Could you check a few things on this model? Use its own coordinates, in mm. A direction names the side the tool comes from. Give positions to 0.01 mm unless a question says otherwise; leave off trailing zeros. Loops run counter-clockwise (first coordinate to the right, second up) from the corner with the lowest first, then second, coordinate; pieces in that order, holes last.
1. Imagine slicing it at A-A (x = 0). List the corners of the cut face in (y, z) for me.
2. Imagine slicing it at C-C (z = 25). List the corners of the cut face in (x, y) for me.
3. Imagine slicing it at B-B (y = 3.5). List the corners of the cut face in (x, z) for me, plus the area to 3 significant figures.
4. Thinking about a two-plate mould opening in Z: for faces 1 (the cylindrical face through (14.531, 8.972, -15.846)), 2 (the cylindrical face through (-27.53, 4.82, -0.33)), 3 (the flat face through (-17.4, 11, 3.1)), which applies, +Z half, -Z half, draft (parallel to the pull), parting line (faces both ways), or undercut?
5. For P1, Ø6.5, axis at x = -25, z = 0, coming from the +Y side; P2, Ø21, axis at x = 0, z = 0, coming from the +Y side; P3, Ø5, axis at x = 17.5, z = 18, coming from the -Y side; P4, Ø6, axis at x = -11, y = 1.5, coming from the +Z side, each with a flat end and sliding along its axis, tell me the tip position at first contact or that it passes through.
6. I need wall thicknesses on line 1 along X through (y, z) = (5.75, 0); line 2 along X through (y, z) = (8.5, 0); line 3 along Y through (x, z) = (13, -19). Which ranges of each line are inside material? Lowest first, please.
7. Imagine slicing it at D-D (x = -11). List the corners of the cut face in (y, z) for me.
8. For faces 4 (the flat face through (-9, 7, 20)), 5 (the cylindrical face through (27.53, 4.82, 0.33)), which set-ups out of +Z, -Z, +X, -X, +Y, -Y let a thin tool reach every point of the face, with its end or its side?
```python
from build123d import *

# Parameters (mm, degrees)
SKETCH1_R                    = 30
SKETCH1_R_2                  = 17.5
BOSS_EXTRUDE1_DEPTH          = 7
SKETCH2_R                    = 21.5
SKETCH2_R_2                  = 17.5
BOSS_EXTRUDE2_DEPTH          = 4
SKETCH4_R                    = 2.55
CUT_EXTRUDE1_DEPTH           = 44.829214002
CHAMFER1_SIZE                = 2.7
CIRPATTERN1_COUNT            = 4
CHAMFER1_OF_CIRPATTERN1_SIZE = 2.7


with BuildPart() as part:
    # Sketch1 → Boss-Extrude1 (new body)
    with BuildSketch(Plane(origin=(0, 0, 0), x_dir=(1, 0, 0), z_dir=(0, 1, 0))):
        with Locations(Location((0, 0, 0), (0, 0, 270))):
            Circle(SKETCH1_R)
        with Locations(Location((0, 0, 0), (0, 0, 270))):
            Circle(SKETCH1_R_2, mode=Mode.SUBTRACT)
    extrude(amount=BOSS_EXTRUDE1_DEPTH)

    # Sketch2 → Boss-Extrude2 (add)
    with BuildSketch(Plane(origin=(0, 7, 0), x_dir=(1, 0, 0), z_dir=(0, 1, 0))):
        with Locations(Location((0, 0, 0), (0, 0, 270))):
            Circle(SKETCH2_R)
        with Locations(Location((0, 0, 0), (0, 0, 270))):
            Circle(SKETCH2_R_2, mode=Mode.SUBTRACT)
    extrude(amount=BOSS_EXTRUDE2_DEPTH)

    # Sketch4 → Cut-Extrude1 (cut, through all)
    with BuildSketch(Plane.XZ):
        with Locations(Location((25, 0, 0), (0, 0, 270))):
            Circle(SKETCH4_R)
    cut_extrude1 = extrude(amount=-CUT_EXTRUDE1_DEPTH, mode=Mode.SUBTRACT)

    # Chamfer1
    # the kernel refuses this chamfer: 2.7 mm, written as the material it takes off along each edge
    with BuildSketch(Plane(origin=(25, 0, 0), x_dir=(0, 0, -1), z_dir=(-1, 0, 0))) as chamfer1_piece_1:
        Polygon((2.55 + CHAMFER1_SIZE, 0), (2.55, -CHAMFER1_SIZE), (2.55, 0), align=None)
    revolve(axis=Axis((25, 0, 0), (0, -1, 0)), mode=Mode.SUBTRACT)

    # CirPattern1: Cut-Extrude1 ×4 about axis
    cirpattern1_axis = Axis((0, 0, 0), (0, 1, 0))
    for i in range(1, CIRPATTERN1_COUNT):
        add(cut_extrude1.rotate(cirpattern1_axis, i * 360 / CIRPATTERN1_COUNT), mode=Mode.SUBTRACT)

    # Chamfer1 of CirPattern1
    # the kernel refuses this chamfer: 2.7 mm, written as the material it takes off along each edge
    with BuildSketch(Plane(origin=(0, 0, -25), x_dir=(-1, 0, 0), z_dir=(0, 0, 1))) as chamfer1_of_cirpattern1_piece_1:
        Polygon((2.55 + CHAMFER1_OF_CIRPATTERN1_SIZE, 0), (2.55, -CHAMFER1_OF_CIRPATTERN1_SIZE), (2.55, 0), align=None)
    revolve(axis=Axis((0, 0, -25), (0, -1, 0)), mode=Mode.SUBTRACT)
    with BuildSketch(Plane(origin=(-25, 0, 0), x_dir=(0, 0, 1), z_dir=(1, 0, 0))) as chamfer1_of_cirpattern1_piece_2:
        Polygon((2.55 + CHAMFER1_OF_CIRPATTERN1_SIZE, 0), (2.55, -CHAMFER1_OF_CIRPATTERN1_SIZE), (2.55, 0), align=None)
    revolve(axis=Axis((-25, 0, 0), (0, -1, 0)), mode=Mode.SUBTRACT)
    with BuildSketch(Plane(origin=(0, 0, 25), x_dir=(1, 0, 0), z_dir=(0, 0, -1))) as chamfer1_of_cirpattern1_piece_3:
        Polygon((2.55 + CHAMFER1_OF_CIRPATTERN1_SIZE, 0), (2.55, -CHAMFER1_OF_CIRPATTERN1_SIZE), (2.55, 0), align=None)
    revolve(axis=Axis((0, 0, 25), (0, -1, 0)), mode=Mode.SUBTRACT)


solid = part.part
```
Derived:
1. outline: (0, -19.75) - (2.7, -22.45) - (7, -22.45) - (7, -21.5) - (11, -21.5) - (11, -17.5) - (0, -17.5) - close; (0, 17.5) - (11, 17.5) - (11, 21.5) - (7, 21.5) - (7, 22.45) - (2.7, 22.45) - (0, 19.75) - close; (0.25, -30) - (7, -30) - (7, -27.55) - (2.7, -27.55) - close; (0.25, 30) - (2.7, 27.55) - (7, 27.55) - (7, 30) - close
2. outline: (-16.58, 0) - (-5.25, 0) - (-2.55, 2.7) - (-2.55, 7) - (-16.58, 7) - close; (2.55, 2.7) - (5.25, 0) - (16.58, 0) - (16.58, 7) - (2.55, 7) - close
3. outline: circle Ø60 at (0, 0); hole circle Ø5.1 at (-25, 0); hole circle Ø35 at (0, 0); hole circle Ø5.1 at (0, -25); hole circle Ø5.1 at (0, 25); hole circle Ø5.1 at (25, 0)
3. area: 1,780 mm2
4. face 1: parting line
4. face 2: undercut
4. face 3: draft
5. P1: stops at y = 7
5. P2: passes through
5. P3: stops at y = 0
5. P4: stops at z = 28.91
6. line 1: x = -30 to -27.55, -22.45 to -17.5, 17.5 to 22.45, 27.55 to 30
6. line 2: x = -21.5 to -17.5, 17.5 to 21.5
6. line 3: y = 0 to 7
7. outline: (0, -27.91) - (7, -27.91) - (7, -18.47) - (11, -18.47) - (11, -13.61) - (0, -13.61) - close; (0, 13.61) - (11, 13.61) - (11, 18.47) - (7, 18.47) - (7, 27.91) - (0, 27.91) - close
8. face 4: +Y
8. face 5: +Y, -Y
